Can you work these out from the model? Positions are in its coordinate system, mm. A direction names the side the tool comes from. Round coordinates to 2 decimals unless told otherwise and drop trailing zeros. Write each loop counter-clockwise with the first axis right and the second up, starting at its lowest first coordinate (ties: lowest second). Pieces come first, ordered by that corner, then holes.
Q1. If we section it at B-B (x = 0): Please give me the cut outline in (y, z).
Q2. If we section it at C-C (z = 0): Please give me the cut outline in (x, y).
Q3. If we section it at A-A (y = 7.5): Give the number of separate pieces and of enclosed holes in the cut face, plus the area to 3 significant figures.
Q4. If we section it at D-D (x = -8): Please give me the cut outline in (y, z), plus the area to 3 significant figures.
Q5. We'd pull the mould along X, two halves only. Please class faces 1 (the cylindrical face through (20.414, 8.327, 0.208)), 2 (the flat face through (20, 16, -8)), 3 (the cylindrical face through (-21.9, 1.52, -21.93)): +X half, -X half, draft (parallel to the pull), parting line (faces both ways), or undercut.
Q6. Please list where these lines run through material, in increasing order: line 1 along Z through (x, y) = (-18, 0.35); line 2 along X through (y, z) = (13.5, -7); line 3 along X through (y, z) = (7.95, 0).
Q7. I'm going to push flat-ended pins straight in: pin 1 Ø2.5 at (x, z) = (18, -18) entering from -Y; pin 2 Ø6.5 at (x, z) = (-16.5, 17) entering from +Y; pin 3 Ø6 at (x, y) = (-19, 8) entering from -Z; pin 4 Ø2.5 at (x, y) = (-6.5, 12) entering from +Z. Where does each tip first touch, or does it pass through?
Q8. For faces 4 (the flat face through (8, 13, 21.9)), 5 (the flat face through (20.65, 2.14, 18.73)), 6 (the flat face through (8, 13, -21.9)), 7 (the flat face through (0, 8, 18)), 8 (the flat face through (22.5, 1, 16)), which set-ups out of +Z, -Z, +X, -X, +Y, -Y let a thin tool reach every point of the face, with its end or its side?
from build123d import *

# Parameters (mm, degrees)
SKETCH1_W                                      = 30
SKETCH1_H                                      = 30
BOSS_EXTRUDE1_DEPTH                            = 3
SKETCH2_W                                      = 20
SKETCH2_H                                      = 7
SKETCH2_W_2                                    = 7
SKETCH2_H_2                                    = 20
BOSS_EXTRUDE2_DEPTH                            = 7
SKETCH3_W                                      = 4.875
SKETCH3_H                                      = 3.9
SKETCH3_W_2                                    = 3.9
SKETCH3_H_2                                    = 4.875
BOSS_EXTRUDE3_DEPTH                            = 6
CSK_FOR_M3_FLAT_HEAD_MACHINE_SCREW1_AT_2_COUNT = 2
CSK_FOR_M3_FLAT_HEAD_MACHINE_SCREW1_AT_2_PITCH = 31.112698372
CSK_FOR_M3_FLAT_HEAD_MACHINE_SCREW1_AT_3_COUNT = 2
CSK_FOR_M3_FLAT_HEAD_MACHINE_SCREW1_AT_3_PITCH = 44
CSK_FOR_M3_FLAT_HEAD_MACHINE_SCREW1_AT_4_COUNT = 2
CSK_FOR_M3_FLAT_HEAD_MACHINE_SCREW1_AT_4_PITCH = 31.112698372
CSK_FOR_M3_FLAT_HEAD_MACHINE_SCREW1_AT_5_COUNT = 2
CSK_FOR_M3_FLAT_HEAD_MACHINE_SCREW1_AT_5_PITCH = 22
CUT_EXTRUDE1_DEPTH                             = 1.75
SKETCH7_R                                      = 1.55
CUT_EXTRUDE2_DEPTH                             = 4
FILLET1_R                                      = 2
SKETCH8_W                                      = 10
SKETCH8_H                                      = 10
CUT_EXTRUDE3_DEPTH                             = 5
SKETCH11_R                                     = 0.8
CUT_EXTRUDE4_DEPTH                             = 7


with BuildPart() as part:
    # Sketch1 → Boss-Extrude1 (new body)
    with BuildSketch(Plane(origin=(0, 0, 0), x_dir=(1, 0, 0), z_dir=(0, 1, 0))):
        Polygon((-10, 22.5), (-10, 25), (10, 25), (10, 22.5), (22.5, 22.5), (22.5, 10), (25, 10), (25, -10), (22.5, -10), (22.5, -22.5), (10, -22.5), (10, -25), (-10, -25), (-10, -22.5), (-22.5, -22.5), (-22.5, -10), (-25, -10), (-25, 10), (-22.5, 10), (-22.5, 22.5), align=None)
        Rectangle(SKETCH1_W, SKETCH1_H, mode=Mode.SUBTRACT)
    extrude(amount=BOSS_EXTRUDE1_DEPTH)

    # Sketch2 → Boss-Extrude2 (add)
    with BuildSketch(Plane(origin=(0, 3, 0), x_dir=(1, 0, 0), z_dir=(0, 1, 0))):
        with Locations((0, 21.5)):
            Rectangle(SKETCH2_W, SKETCH2_H)
        with Locations((21.5, 0)):
            Rectangle(SKETCH2_W_2, SKETCH2_H_2)
        with Locations((0, -21.5)):
            Rectangle(SKETCH2_W, SKETCH2_H)
        with Locations((-21.5, 0)):
            Rectangle(SKETCH2_W_2, SKETCH2_H_2)
    extrude(amount=BOSS_EXTRUDE2_DEPTH)

    # Sketch3 → Boss-Extrude3 (add)
    with BuildSketch(Plane(origin=(0, 10, 0), x_dir=(1, 0, 0), z_dir=(0, 1, 0))):
        with Locations((-7.5625, 19.95)):
            Rectangle(SKETCH3_W, SKETCH3_H)
        with Locations((7.5625, 19.95)):
            Rectangle(SKETCH3_W, SKETCH3_H)
        with Locations((19.95, 7.5625)):
            Rectangle(SKETCH3_W_2, SKETCH3_H_2)
        with Locations((19.95, -7.5625)):
            Rectangle(SKETCH3_W_2, SKETCH3_H_2)
        with Locations((7.5625, -19.95)):
            Rectangle(SKETCH3_W, SKETCH3_H)
        with Locations((-7.5625, -19.95)):
            Rectangle(SKETCH3_W, SKETCH3_H)
        with Locations((-19.95, -7.5625)):
            Rectangle(SKETCH3_W_2, SKETCH3_H_2)
        with Locations((-19.95, 7.5625)):
            Rectangle(SKETCH3_W_2, SKETCH3_H_2)
    extrude(amount=BOSS_EXTRUDE3_DEPTH)

    # Sketch4 → CSK for M3 Flat Head Machine Screw1 (revolve, cut)
    with BuildSketch(Plane(origin=(-22, 0, 0), x_dir=(0, 0, -1), z_dir=(1, 0, 0))):
        Polygon((0, 0), (0, 20.96137699), (1.6, 20), (1.6, 1.7), (3.15, 0.15), (3.15, 0), align=None)
    csk_for_m3_flat_head_machine_screw1 = revolve(axis=Axis((-22, -6.35, 0), (0, 1, 0)), mode=Mode.SUBTRACT)

    # CSK for M3 Flat Head Machine Screw1 at 2: CSK for M3 Flat Head Machine Screw1 ×2
    with Locations(*[Vector(0.707106781, 0, 0.707106781) * (i * CSK_FOR_M3_FLAT_HEAD_MACHINE_SCREW1_AT_2_PITCH) for i in range(1, CSK_FOR_M3_FLAT_HEAD_MACHINE_SCREW1_AT_2_COUNT)]):
        add(csk_for_m3_flat_head_machine_screw1, mode=Mode.SUBTRACT)

    # CSK for M3 Flat Head Machine Screw1 at 3: CSK for M3 Flat Head Machine Screw1 ×2
    with Locations(*[(i * CSK_FOR_M3_FLAT_HEAD_MACHINE_SCREW1_AT_3_PITCH, 0, 0) for i in range(1, CSK_FOR_M3_FLAT_HEAD_MACHINE_SCREW1_AT_3_COUNT)]):
        add(csk_for_m3_flat_head_machine_screw1, mode=Mode.SUBTRACT)

    # CSK for M3 Flat Head Machine Screw1 at 4: CSK for M3 Flat Head Machine Screw1 ×2
    with Locations(*[Vector(0.707106781, 0, -0.707106781) * (i * CSK_FOR_M3_FLAT_HEAD_MACHINE_SCREW1_AT_4_PITCH) for i in range(1, CSK_FOR_M3_FLAT_HEAD_MACHINE_SCREW1_AT_4_COUNT)]):
        add(csk_for_m3_flat_head_machine_screw1, mode=Mode.SUBTRACT)

    # CSK for M3 Flat Head Machine Screw1 at 5: CSK for M3 Flat Head Machine Screw1 ×2
    with Locations(*[(i * CSK_FOR_M3_FLAT_HEAD_MACHINE_SCREW1_AT_5_PITCH, 0, 0) for i in range(1, CSK_FOR_M3_FLAT_HEAD_MACHINE_SCREW1_AT_5_COUNT)]):
        add(csk_for_m3_flat_head_machine_screw1, mode=Mode.SUBTRACT)

    # Sketch6 → Cut-Extrude1 (cut)
    with BuildSketch(Plane(origin=(0, 3, 0), x_dir=(1, 0, 0), z_dir=(0, 1, 0))):
        Polygon((-20.245365598, 20.245365598), (-21.067226447, 17.178139151), (-18.821860849, 14.932773553), (-15.754634402, 15.754634402), (-14.932773553, 18.821860849), (-17.178139151, 21.067226447), align=None)
        Polygon((20.245365598, 20.245365598), (17.178139151, 21.067226447), (14.932773553, 18.821860849), (15.754634402, 15.754634402), (18.821860849, 14.932773553), (21.067226447, 17.178139151), align=None)
        Polygon((20.245365598, -20.245365598), (21.067226447, -17.178139151), (18.821860849, -14.932773553), (15.754634402, -15.754634402), (14.932773553, -18.821860849), (17.178139151, -21.067226447), align=None)
        Polygon((-20.245365598, -20.245365598), (-17.178139151, -21.067226447), (-14.932773553, -18.821860849), (-15.754634402, -15.754634402), (-18.821860849, -14.932773553), (-21.067226447, -17.178139151), align=None)
    extrude(amount=-CUT_EXTRUDE1_DEPTH, mode=Mode.SUBTRACT)

    # Sketch7 → Cut-Extrude2 (cut, through all)
    with BuildSketch(Plane(origin=(0, 3, 0), x_dir=(1, 0, 0), z_dir=(0, 1, 0))):
        with Locations((-18, 18)):
            Circle(SKETCH7_R)
        with Locations((18, 18)):
            Circle(SKETCH7_R)
        with Locations((18, -18)):
            Circle(SKETCH7_R)
        with Locations((-18, -18)):
            Circle(SKETCH7_R)
    extrude(amount=-CUT_EXTRUDE2_DEPTH, mode=Mode.SUBTRACT)

    # Fillet1
    fillet1_edges = [part.edges().sort_by_distance(p)[0] for p in [
        (-15, 1.5, -15),
        (-15, 1.5, 15),
        (15, 1.5, 15),
        (15, 1.5, -15),
        (-10, 1.5, -22.5),
        (-22.5, 1.5, -10),
        (10, 1.5, -22.5),
        (22.5, 1.5, -10),
        (22.5, 1.5, 10),
        (10, 1.5, 22.5),
        (-10, 1.5, 22.5),
        (-22.5, 1.5, 10),
        (-22.5, 1.5, 22.5),
        (22.5, 1.5, 22.5),
        (22.5, 1.5, -22.5),
        (-22.5, 1.5, -22.5),
    ]]
    fillet(fillet1_edges, radius=FILLET1_R)

    # Sketch8 → Cut-Extrude3 (cut)
    with BuildSketch(Plane.XZ):
        with Locations((20, 0)):
            Rectangle(SKETCH8_W, SKETCH8_H)
    extrude(amount=-CUT_EXTRUDE3_DEPTH, mode=Mode.SUBTRACT)

    # Sketch9 → CSK for M3 Flat Head Machine Screw2 (revolve, cut)
    with BuildSketch(Plane(origin=(22, 5, 0), x_dir=(0, 0, -1), z_dir=(1, 0, 0))):
        Polygon((0, 0), (0, 20.96137699), (1.6, 20), (1.6, 1.7), (3.15, 0.15), (3.15, 0), align=None)
    revolve(axis=Axis((22, -1.35, 0), (0, 1, 0)), mode=Mode.SUBTRACT)

    # Sketch11 → Cut-Extrude4 (cut)
    with BuildSketch(Plane(origin=(25, 0, 0), x_dir=(0, 0, -1), z_dir=(1, 0, 0))):
        with Locations((7, 7.5)):
            Circle(SKETCH11_R)
        with Locations((-7, 7.5)):
            Circle(SKETCH11_R)
    extrude(amount=-CUT_EXTRUDE4_DEPTH, mode=Mode.SUBTRACT)


solid = part.part
A:
1. outline: (0, -18.85) - (0.15, -18.85) - (1.7, -20.4) - (10, -20.4) - (10, -18) - (3, -18) - (3, -15) - (0, -15) - close; (0, 15) - (3, 15) - (3, 18) - (10, 18) - (10, 20.4) - (1.7, 20.4) - (0.15, 18.85) - (0, 18.85) - close; (0.3, -25) - (10, -25) - (10, -23.6) - (1.7, -23.6) - close; (0.3, 25) - (1.7, 23.6) - (10, 23.6) - (10, 25) - close
2. outline: (-25, 0.3) - (-23.6, 1.7) - (-23.6, 10) - (-25, 10) - close; (-20.4, 1.7) - (-18.85, 0.15) - (-18.85, 0) - (-15, 0) - (-15, 3) - (-18, 3) - (-18, 10) - (-20.4, 10) - close; (18, 5) - (18.85, 5) - (18.85, 5.15) - (20.4, 6.7) - (20.4, 10) - (18, 10) - close; (23.6, 6.7) - (25, 5.3) - (25, 10) - (23.6, 10) - close
3. separate pieces: 6
3. enclosed holes: 4
3. area: 505 mm2
4. outline: (0, -25) - (10, -25) - (10, -21.9) - (16, -21.9) - (16, -18) - (3, -18) - (3, -15) - (0, -15) - close; (0, 15) - (3, 15) - (3, 18) - (16, 18) - (16, 21.9) - (10, 21.9) - (10, 25) - (0, 25) - close
4. area: 205 mm2
5. face 1: undercut
5. face 2: draft
5. face 3: -X half
6. line 1: z = -22.5 to -19.55, -16.45 to 16.45, 19.55 to 22.5
6. line 2: x = -21.9 to -18, 18 to 21.9
6. line 3: x = -25 to -23.6, -20.4 to -18, 18 to 20.4, 23.6 to 25
7. pin 1: passes through
7. pin 2: stops at y = 3
7. pin 3: stops at z = -10
7. pin 4: stops at z = 21.9
8. face 4: +Z, +X, -X, +Y
8. face 5: +Y
8. face 6: -Z, +X, -X, +Y
8. face 7: +X, -X, +Y
8. face 8: +Z, +X, +Y, -Y
